Part model, mm, in its own coordinate system. Round coordinates to 2 decimals unless told otherwise and drop trailing zeros. Loops run counter-clockwise (first coordinate to the right, second up) from the corner with the lowest first, then second, coordinate; pieces in that order, holes last. Notation, with made-up numbers: M -36,40 L 19,40 A16 ccw 19,44 Z; hole C 89.5,55 d11. An arc over 180 degrees is marked long. Put each result on its own line as item: value. Start each with the question number.
1) Slice it at A-A on z = 164. Give the cut face in (x, y), then the cut area to 3 significant figures.
2) Pull direction X, two halves, no side cores. Call faces 1 (the flat face through (0, 2, 99.06)), 2 (the cylindrical face through (-7.559, -5.796, 48.872)): +X half, -X half, draft (parallel to the pull), parting line (faces both ways), or undercut.
3) Probe line 1 along Z through (x, y) = (-4.5, 1); line 2 along X through (y, z) = (-0.5, 58); line 3 along Z through (x, y) = (3, 6.75). List the from-to ranges inside material, lowest first.
4) Drop flat-ended pins along their axis: pin 1 Ø8 at (y, z) = (4.5, 109) entering from -X; pin 2 Ø10 at (y, z) = (0.5, 165) entering from +X; pin 3 Ø4 at (x, z) = (-4, 100.5) entering from -Y. Give the stop position or say it passes through.
```python
from build123d import *

# Parameters (mm, degrees)
F0_R     = 9.525
F1_DEPTH = 99.06
F2_R     = 1.4605
F3_DEPTH = 101.6
F4_R     = 0.635
F5_R     = 2.54
F6_R     = 2.54


with BuildPart() as f1:
    # F0 (on Top) → F1 (new body)
    with BuildSketch(Plane.XY):
        Circle(F0_R)
    extrude(amount=F1_DEPTH)

    # F2 (on face) → F3 (join)
    with BuildSketch(Plane.XY.offset(99.06)):
        Circle(F2_R)
    extrude(amount=F3_DEPTH)

    # F4
    f4_edges = [f1.edges().sort_by_distance(p)[0] for p in [
        (-1.4605, 0, 200.66),
    ]]
    fillet(f4_edges, radius=F4_R)

    # F5
    f5_edges = [f1.edges().sort_by_distance(p)[0] for p in [
        (-9.525, 0, 0),
    ]]
    fillet(f5_edges, radius=F5_R)

    # F6
    f6_edges = [f1.edges().sort_by_distance(p)[0] for p in [
        (-9.525, 0, 99.06),
    ]]
    fillet(f6_edges, radius=F6_R)


solid = f1.part
```
Recorded:
1. outline: C 0,0 d2.92
1. area: 6.70 mm2
2. face 1: draft
2. face 2: parting line
3. line 1: z = 0 to 99.06
3. line 2: x = -9.51 to 9.51
3. line 3: z = 0.03 to 99.03
4. pin 1: stops at x = -1.37
4. pin 2: stops at x = 1.46
4. pin 3: stops at y = -7.74
